from build123d import *

# Parameters (mm, degrees)
F0_W     = 46
F0_H     = 76
F1_DEPTH = 3
F2_W     = 46
F2_H     = 76
F2_W_2   = 40
F2_H_2   = 70
F3_DEPTH = 15
F5_DEPTH = 25
F6_W     = 40
F6_H     = 42
F7_DEPTH = 3
F8_DEPTH = 25


with BuildPart() as f1:
    # F0 (on Top) → F1 (new body)
    with BuildSketch(Plane.XY):
        Rectangle(F0_W, F0_H)
    extrude(amount=F1_DEPTH)

    # F2 (on face) → F3 (join)
    with BuildSketch(Plane.XY.offset(3)):
        Rectangle(F2_W, F2_H)
        Rectangle(F2_W_2, F2_H_2, mode=Mode.SUBTRACT)
    extrude(amount=F3_DEPTH)

    # F4 (on face) → F5 (cut)
    with BuildSketch(Plane.XY.offset(3)):
        with BuildLine():
            Line((-10, 28), (-7.0000000819, 28))
            ThreePointArc((-7, 28), (-4, 31.000000041), (-7.0000000819, 34))
            Line((-7.0000000819, 34), (-10, 34))
            ThreePointArc((-10, 34), (-13, 31), (-10, 28))
        make_face()
        with BuildLine():
            Line((10, 34), (7, 34))
            ThreePointArc((7, 34), (4, 31), (7, 28))
            Line((7, 28), (10, 28))
            ThreePointArc((10, 28), (13, 31), (10, 34))
        make_face()
    extrude(amount=-F5_DEPTH, mode=Mode.SUBTRACT)

    # F6 (on face) → F7 (join)
    with BuildSketch(Plane.XY.offset(18)):
        Polygon((-23, 7), (-23, -38), (23, -38), (23, 7), (20, 7), (20, -35), (-20, -35), (-20, 7), align=None)
        with Locations((0, -14)):
            Rectangle(F6_W, F6_H)
    extrude(amount=F7_DEPTH)

    # F8 (cut): a face of the model
    f8_faces = [f1.faces().sort_by_distance(p)[0] for p in [
        (0, 35, 10.5),
    ]]
    extrude(f8_faces, amount=-F8_DEPTH, mode=Mode.SUBTRACT)


solid = f1.part
Work out the finished part from the listing and answer in its coordinate system (mm). A direction names the side the tool comes from. Give positions to 0.01 mm unless a question says otherwise; leave off trailing zeros. Loops run counter-clockwise (first coordinate to the right, second up) from the corner with the lowest first, then second, coordinate; pieces in that order, holes last. Notation, with made-up numbers: (17, 55) - (51, 55) arc R23 ccw to (51, 83) - close; hole circle Ø10 at (-18, -16.5). An arc over 180 degrees is marked (long way). Answer in a Markdown table with one row per item. Add a question column.
Q1. Consider line 1 along X through (y, z) = (-18.5, 13.5); line 2 along Z through (x, y) = (-11, -29); line 3 along Z through (x, y) = (19.5, 25). Determine where each line is inside the solid, lowest interval first.
Q2. Each of these flat-tipped pins is pushed along its axis until it touches: P1, Ø12, axis at x = -3, z = 10.5, coming from the +Y side; P2, Ø3.5, axis at x = 8.5, z = 19, coming from the +Y side; P3, Ø8, axis at x = -12.5, y = -29.5, coming from the -Z side; P4, Ø10, axis at x = -4, y = 21, coming from the +Z side. Where does it stop, or does it pass through?
Q3. The part is cut by section A-A (y = 31). Determine the outline of the cut face in (x, z).
Q4. The part is cut by section B-B (y = 6). Determine the outline of the cut face in (x, z), and give its area (3 significant figures).
Q5. A tool of negligible diameter and unlimited length cuts with its end or side. For faces 5 (the flat face through (0, 38, 1)), 6 (the cylindrical face through (-4, 31, 2)), 7 (the flat face through (21, 23, 18)), 8 (the flat face through (0, 1, 3)), 9 (the flat face through (0, -15, 21)), from which of +Z, -Z, +X, -X, +Y, -Y can it reach the whole face along a straight path? Write none if from no direction.
Q6. The part is cut by section C-C (z = 15.25). Determine the outline of the cut face in (x, y).
Q7. The part is cut by section D-D (x = -11). Determine the outline of the cut face in (y, z), and give its area (3 significant figures).
Q8. Determine the mould class of faces 1 (the flat face through (-20, 1, 10)), 2 (the flat face through (0, 7, 19)), 3 (the flat face through (8, 28, 2)), 4 (the flat face through (-9, 28, 2)) for opening direction Y: released by +Y, released by -Y, zero draft, split by the parting line, or undercut.
Solution:
| question | item | result |
|---|---|---|
| 1 | line 1 | x = -23 to -20, 20 to 23 |
| 1 | line 2 | z = 0 to 3, 18 to 21 |
| 1 | line 3 | z = 0 to 3 |
| 2 | P1 | stops at y = -35 |
| 2 | P2 | stops at y = 7 |
| 2 | P3 | stops at z = 0 |
| 2 | P4 | stops at z = 3 |
| 3 | outline | (-23, 0) - (-13, 0) - (-13, 3) - (-20, 3) - (-20, 18) - (-23, 18) - close; (-4, 0) - (4, 0) - (4, 3) - (-4, 3) - close; (13, 0) - (23, 0) - (23, 18) - (20, 18) - (20, 3) - (13, 3) - close |
| 4 | outline | (-23, 0) - (23, 0) - (23, 21) - (-23, 21) - close; hole (-20, 3) - (20, 3) - (20, 18) - (-20, 18) - close |
| 4 | area | 366 mm² |
| 5 | face 5 | +Z, -Z, +X, -X, +Y |
| 5 | face 6 | +Z, -Z |
| 5 | face 7 | +Z, +X, -X, +Y |
| 5 | face 8 | +Y |
| 5 | face 9 | +Z, +X, -X, +Y, -Y |
| 6 | outline | (-23, -38) - (23, -38) - (23, 38) - (20, 38) - (20, -35) - (-20, -35) - (-20, 38) - (-23, 38) - close |
| 7 | outline | (-38, 0) - (28.17, 0) - (28.17, 3) - (-35, 3) - (-35, 18) - (7, 18) - (7, 21) - (-38, 21) - close; (33.83, 0) - (38, 0) - (38, 3) - (33.83, 3) - close |
| 7 | area | 391 mm² |
| 8 | face 1 | zero draft |
| 8 | face 2 | released by +Y |
| 8 | face 3 | undercut |
| 8 | face 4 | undercut |
